```python
from build123d import *

# Parameters (mm, degrees)
BOSS_EXTRUDE1_DEPTH = 150
SKETCH3_R           = 1.5
CUT_EXTRUDE1_DEPTH  = 5
LPATTERN1_COUNT     = 36
LPATTERN1_PITCH     = 4


with BuildPart() as part:
    # Sketch2 → Boss-Extrude1 (new body)
    with BuildSketch(Plane(origin=(0, 0, 0), x_dir=(0, 0, -1), z_dir=(1, 0, 0))):
        Polygon((-7, -1.5), (7, -1.5), (7, 1.5), (5.5, 1.5), (5.5, -1), (0, 0.5), (-5.5, -1), (-5.5, 1.5), (-7, 1.5), align=None)
    extrude(amount=BOSS_EXTRUDE1_DEPTH)

    # Sketch3 → Cut-Extrude1 (cut)
    with BuildSketch(Plane.XZ.offset(1.5)):
        with Locations(Location((5, 0, 0), (0, 0, 270))):
            Circle(SKETCH3_R)
    cut_extrude1 = extrude(amount=-CUT_EXTRUDE1_DEPTH, mode=Mode.SUBTRACT)

    # LPattern1: Cut-Extrude1 ×36
    with Locations(*[(i * LPATTERN1_PITCH, 0, 0) for i in range(1, LPATTERN1_COUNT)]):
        add(cut_extrude1, mode=Mode.SUBTRACT)


solid = part.part
```
Work out the finished part from the listing and answer in its coordinate system (mm). A direction names the side the tool comes from. Round coordinates to 2 decimals unless told otherwise and drop trailing zeros. Write each loop counter-clockwise with the first axis right and the second up, starting at its lowest first coordinate (ties: lowest second). Pieces come first, ordered by that corner, then holes.
1) Which of the six approach directions +Z, -Z, +X, -X, +Y, -Y give full straight-line access (tool end or side, diameter ignored) to faces 4 (the face through (53.07, -0.74, 1.5)), 5 (the face through (73.95, -0.427, -3.4))?
2) Flat-ended cylindrical pins translate along their axes: P1, Ø1.5, axis at x = 121.5, z = 3.5, coming from the +Y side; P2, Ø4, axis at x = 25, z = 0, coming from the +Y side. Find the tip coordinate at first contact, or state that the pin passes through.
3) A cutting plane is placed at B-B on z = -4. Determine the outline of the cut face in (x, y), and give its area (3 significant figures).
4) Consider probe 1 along Z at (x, y) = (105.5, 0.7); probe 2 along Z at (x, y) = (144.5, -1.05); probe 3 along Y at (x, z) = (125, -2.5). Determine where each line is inside the solid, lowest interval first.
5) A cutting plane is placed at A-A on x = 65. Determine the outline of the cut face in (y, z), and give its area (3 significant figures).
6) Determine the mould class of faces 1 (the face through (0, 0, 0)), 2 (the face through (97.07, -0.74, 1.5)), 3 (the face through (74, 0, -7)) for opening direction Z: pulls with the +Z half, pulls with the -Z half, needs draft (parallel to the pull), parting line crosses it, or undercut.
Entries:
1. face 4: +Y, -Y
1. face 5: +X, -X, +Y
2. P1: stops at y = -0.25
2. P2: stops at y = 0.5
3. outline: (0, -1.5) - (150, -1.5) - (150, -0.59) - (0, -0.59) - close
3. area: 136 mm2
4. probe 1: z = -7 to -5.5, 5.5 to 7
4. probe 2: z = -7 to -1.41, 1.41 to 7
4. probe 3: y = -1.5 to -0.18
5. outline: (-1.5, -7) - (1.5, -7) - (1.5, -5.5) - (-1, -5.5) - (0.09, -1.5) - (-1.5, -1.5) - close; (-1.5, 1.5) - (0.09, 1.5) - (-1, 5.5) - (1.5, 5.5) - (1.5, 7) - (-1.5, 7) - close
5. area: 17.4 mm2
6. face 1: needs draft
6. face 2: undercut
6. face 3: pulls with the -Z half
